Design review of the part built by this model. Coordinates are the model's own, in mm. Face numbers are marked on the shaded views. Coordinates: 2 decimals unless noted, no trailing zeros. One line per item, written item: value.
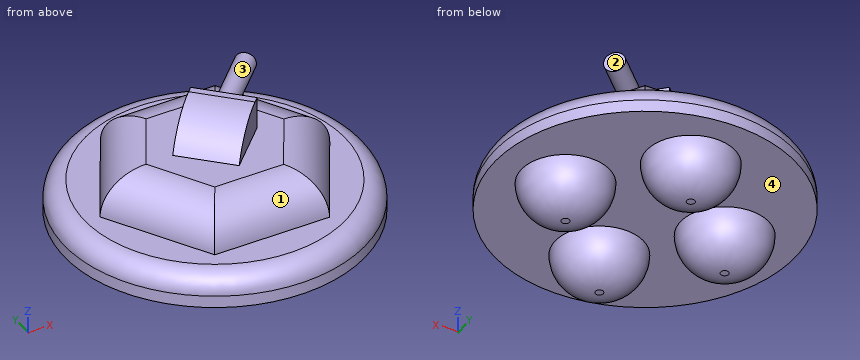
```python
from build123d import *

# Parameters (mm, degrees)
F0_R         = 37.5
F1_DEPTH     = 8
F2_R         = 5
F3_R         = 11
F4_DEPTH     = 10
F5_R         = 9.99999
F7_DEPTH     = 10
F8_R         = 9.99999
F10_DEPTH    = 18
F11_T1_DEPTH = 81.3324958071
F12_R        = 2.5
F13_DEPTH    = 18


# Not quite as in the source:
# - a fillet or chamfer that OpenCascade refuses, or shapes differently, is made with other operations: its cross-section is extruded or revolved along the edge and cut away or added
# - a fillet or chamfer is up to 0.001 mm smaller than in the source, because OpenCascade refuses the exact size


with BuildPart() as f1:
    # F0 (on Top) → F1 (new body)
    with BuildSketch(Plane.XY):
        Circle(F0_R)
    extrude(amount=F1_DEPTH)

    # F2
    f2_edges = [f1.edges().sort_by_distance(p)[0] for p in [
        (-37.5, 0, 8),
    ]]
    fillet(f2_edges, radius=F2_R)

    # F3 (on face) → F4 (join)
    with BuildSketch(Plane(origin=(0, 0, 0), x_dir=(1, 0, 0), z_dir=(0, 0, -1))):
        with Locations((20, 0)):
            Circle(F3_R)
        with Locations((-20, 0)):
            Circle(F3_R)
        with Locations((0, 20)):
            Circle(F3_R)
        with Locations((0, -20)):
            Circle(F3_R)
    extrude(amount=F4_DEPTH)

    # F5 (radius 10 in the source; OpenCascade refuses exactly that, so slightly less here)
    f5_edges = [f1.edges().sort_by_distance(p)[0] for p in [
        (-11, 20, -10),
        (-31, 0, -10),
        (-11, -20, -10),
        (9, 0, -10),
    ]]
    fillet(f5_edges, radius=F5_R)

    # F6 (on face) → F7 (join)
    with BuildSketch(Plane.XY.offset(8)):
        Polygon((14.4337567297, -25), (28.8675134595, 0), (14.4337567297, 25), (-14.4337567297, 25), (-28.8675134595, 0), (-14.4337567297, -25), align=None)
    extrude(amount=F7_DEPTH)

    # F8 (radius 10 in the source; OpenCascade refuses exactly that, so slightly less here)
    f8_edges = [f1.edges().sort_by_distance(p)[0] for p in [
        (0, -25, 18),
        (21.650635, -12.5, 18),
        (21.650635, 12.5, 18),
        (0, 25, 18),
        (-21.650635, 12.5, 18),
        (-21.650635, -12.5, 18),
    ]]
    fillet(f8_edges, radius=F8_R)

    # F9 (on face) → F10 (join)
    with BuildSketch(Plane.XY.offset(8)):
        Polygon((10.6066017178, 0), (0, 10.6066017178), (-10.6066017178, 0), (0, -10.6066017178), align=None)
    extrude(amount=F10_DEPTH)

    # F11: fillet of radius 15 on 1 edges, made by hand

    # F11_s2 → F11_t1 (cut)
    with BuildSketch(Plane(origin=(-28.755379658, 28.755379658, 0), x_dir=(0, 0, 1), z_dir=(0.7071067812, -0.7071067812, 0))):
        with BuildLine():
            ThreePointArc((18, 7.5), (23.8452325787, 1.979467531), (26, -5.7664991614))
            Line((26, -5.7664991614), (26, 7.5))
            Line((26, 7.5), (18, 7.5))
        make_face()
    extrude(amount=F11_T1_DEPTH, mode=Mode.SUBTRACT)

    # F12 (on face) → F13 (join)
    with BuildSketch(Plane(origin=(5.3033008589, 5.3033008589, 0), x_dir=(-0.7071067812, 0.7071067812, 0), z_dir=(0.7071067812, 0.7071067812, 0))):
        with Locations((0, 22)):
            Circle(F12_R)
    extrude(amount=F13_DEPTH)


solid = f1.part
```
(1) To check wall thickness, follow line 1 along Y through (x, z) = (-4, -1); line 2 along Z through (x, y) = (20.5, 19); line 3 along Y through (x, z) = (-8.5, -2). State the ranges of each line that lie inside material, in increasing order. Write a range as [from, to].
Reply:
line 1: y = [-30.19, -9.81], [9.81, 30.19]
line 2: z = [0, 8]
line 3: y = [-26.66, -13.34], [13.34, 26.66]
(2) Mouldability with a two-part tool opening along Z and no side actions: class the marked faces 1, 2, 3 and 4 as released by +Z, released by -Z, zero draft, split by the parting line, or undercut.
Reply:
face 1: released by +Z
face 2: zero draft
face 3: undercut
face 4: released by -Z
(3) Insertion check: pin 1 (6 mm diameter, centred on x = 21, y = 16.5, fed in from +Z); pin 2 (4 mm diameter, centred on x = 4, y = -1.5, fed in from +Z); pin 3 (4 mm diameter, centred on x = 3.5, z = 20.5, fed in from -Y). Each pin has a flat end and moves straight along its axis. Give the tip position at first contact, or say it passes through.
Reply:
pin 1: stops at z = 24.47
pin 2: stops at z = 25.87
pin 3: stops at y = -9.11
